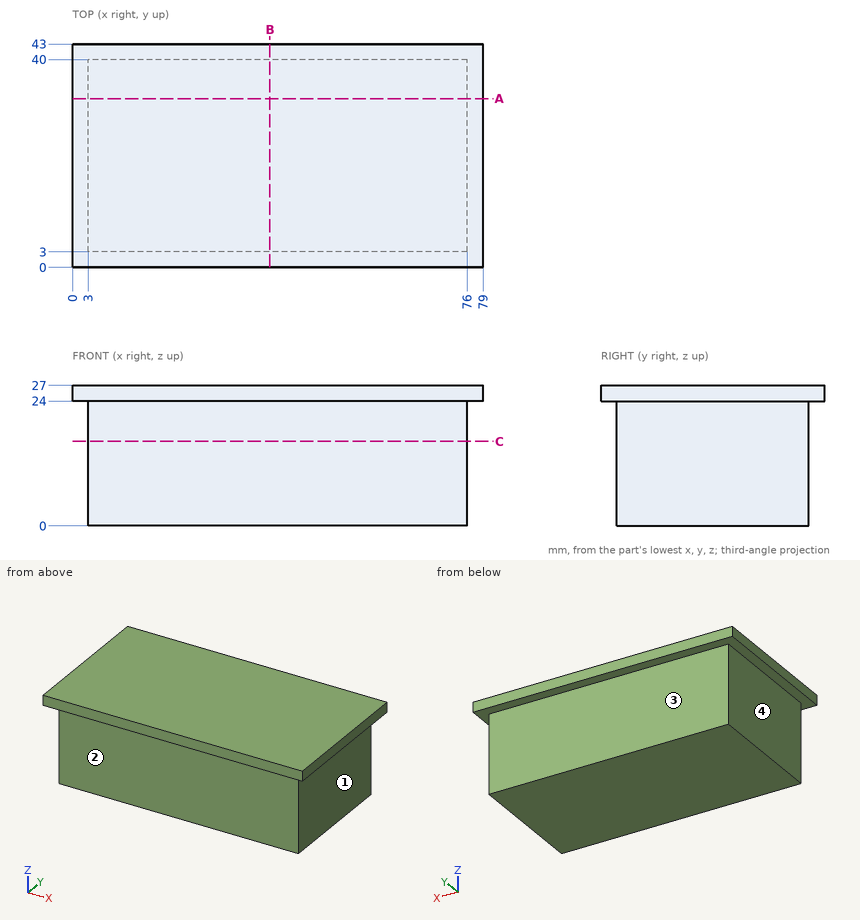
Job drawing, mm, ordinate dimensions from the low corner. One solid piece. A direction names the side the tool comes from. Give positions to 0.01 mm unless a question says otherwise; leave off trailing zeros. Loops run counter-clockwise (first coordinate to the right, second up) from the corner with the lowest first, then second, coordinate; pieces in that order, holes last.
Item 1: Slice it at A-A, the plane y = 32.5. List the corners of the cut face in (x, z), and give its area (3 significant figures).
Answers follow:
outline: (0, 24) - (3, 24) - (3, 0) - (76, 0) - (76, 24) - (79, 24) - (79, 27) - (0, 27) - close
area: 1,990 mm2
Item 2: Slice it at C-C, the plane z = 16.25. List the corners of the cut face in (x, y).
Answers follow:
outline: (3, 3) - (76, 3) - (76, 40) - (3, 40) - close
Item 3: Slice it at B-B, the plane x = 38. List the corners of the cut face in (y, z), and give its area (3 significant figures).
Answers follow:
outline: (0, 24) - (3, 24) - (3, 0) - (40, 0) - (40, 24) - (43, 24) - (43, 27) - (0, 27) - close
area: 1,020 mm2
Item 4: Which spindle directions (+Z, -Z, +X, -X, +Y, -Y) get a long thin tool onto all of the face, cutting with end or side? Do the marked faces 1, 2, 3 and 4. Say none if no direction does.
Answers follow:
face 1: -Z, +X, +Y, -Y
face 2: -Z, +X, -X, -Y
face 3: -Z, +X, -X, +Y
face 4: -Z, -X, +Y, -Y
Item 5: Flat gauge pins, fed straight in: pin 1 (1 mm diameter, centred on y = 21, z = 6.5, fed in from -X); pin 2 (12 mm diameter, centred on y = 26, z = 12.5, fed in from +X); pin 3 (10 mm diameter, centred on x = 45.5, z = 18, fed in from -Y). Where does each tip first touch, or does it go through?
Answers follow:
pin 1: stops at x = 3
pin 2: stops at x = 76
pin 3: stops at y = 3
Item 6: Drill centre lines: line 1 (X direction, y = 6.5, z = 5); line 2 (Y direction, x = 20, z = 10.25). Where is each one in solid material? Low to high.
Answers follow:
line 1: x = 3 to 76
line 2: y = 3 to 40
